from build123d import *

# Parameters (mm, degrees)
SKETCH1_W             = 50
SKETCH1_H             = 50
BOSS_EXTRUDE1_DEPTH   = 10
BOSS_EXTRUDE1_2_DEPTH = 10
BOSS_EXTRUDE2_DEPTH   = 50
SKETCH3_W             = 30
SKETCH3_H             = 30
CUT_EXTRUDE1_DEPTH    = 90
SKETCH4_W             = 10
SKETCH4_H             = 29.860616381
SKETCH4_H_2           = 30
CUT_EXTRUDE2_DEPTH    = 90
SKETCH5_W             = 50
SKETCH5_H             = 50
BOSS_EXTRUDE3_DEPTH   = 10
SKETCH6_R             = 12
CUT_EXTRUDE3_DEPTH    = 80
SKETCH13_W            = 50
SKETCH13_H            = 50
CUT_EXTRUDE5_DEPTH    = 160
SKETCH7_R             = 15.5
BOSS_EXTRUDE4_DEPTH   = 337.81
SKETCH14_W            = 50
SKETCH14_H            = 50
BOSS_EXTRUDE5_DEPTH   = 10
BOSS_EXTRUDE6_DEPTH   = 10
BOSS_EXTRUDE7_DEPTH   = 10
SKETCH17_R            = 15.5
CUT_EXTRUDE6_DEPTH    = 70
SKETCH19_R            = 12.7
CUT_EXTRUDE7_DEPTH    = 70
SKETCH20_R            = 12.7
BOSS_EXTRUDE11_DEPTH  = 10
SKETCH26_R            = 12
BOSS_EXTRUDE12_DEPTH  = 10
SKETCH27_R            = 13
CUT_EXTRUDE8_DEPTH    = 70


with BuildPart() as part:
    # Sketch1 → Boss-Extrude1 (new body)
    with BuildSketch(Plane.XY):
        with Locations((25, 25)):
            Rectangle(SKETCH1_W, SKETCH1_H)
    extrude(amount=BOSS_EXTRUDE1_DEPTH)

    # Sketch2 → Boss-Extrude2 (add)
    with BuildSketch(Plane(origin=(0, 0, 0), x_dir=(1, 0, 0), z_dir=(0, 1, 0))):
        with BuildLine():
            Line((0, 0), (50, 0))
            Line((50, 0), (50, 30))
            ThreePointArc((50, 30), (44.142135624, 44.142135624), (30, 50))
            Line((30, 50), (20, 50))
            ThreePointArc((20, 50), (5.857864376, 44.142135624), (0, 30))
            Line((0, 30), (0, 0))
        make_face()
    extrude(amount=BOSS_EXTRUDE2_DEPTH)

    # Sketch3 → Cut-Extrude1 (cut)
    with BuildSketch(Plane.XY.offset(10)):
        with Locations((25, 25)):
            Rectangle(SKETCH3_W, SKETCH3_H)
    extrude(amount=-CUT_EXTRUDE1_DEPTH, mode=Mode.SUBTRACT)

    # Sketch4 → Cut-Extrude2 (cut)
    with BuildSketch(Plane.XY.offset(10)):
        with Locations((45, 25.06969181)):
            Rectangle(SKETCH4_W, SKETCH4_H)
        with Locations((5, 25)):
            Rectangle(SKETCH4_W, SKETCH4_H_2)
    extrude(amount=-CUT_EXTRUDE2_DEPTH, mode=Mode.SUBTRACT)


with BuildPart() as body_2:
    # Sketch1 → Boss-Extrude1 2 (new body)
    with BuildSketch(Plane.XY):
        with Locations((25, -320)):
            Rectangle(SKETCH1_W, SKETCH1_H)
    extrude(amount=BOSS_EXTRUDE1_2_DEPTH)

    # Sketch13 → Cut-Extrude5 (cut)
    with BuildSketch(Plane(origin=(0, 0, 0), x_dir=(-1, 0, 0), z_dir=(0, 0, -1))):
        with Locations((-25, -320)):
            Rectangle(SKETCH13_W, SKETCH13_H)
    extrude(amount=-CUT_EXTRUDE5_DEPTH, mode=Mode.SUBTRACT)


with BuildPart() as cut_extrude2_piece_1:
    # of the separate pieces the step leaves, piece 1, a body of its own (cut_extrude2_pieces)
    add(part.part.solids().sort_by_distance((0, 0, 10))[0])



with BuildPart() as cut_extrude2_piece_2:
    # of the separate pieces the step leaves, piece 2, a body of its own (cut_extrude2_pieces)
    add(part.part.solids().sort_by_distance((0, 50, 10))[0])


with BuildPart() as cut_extrude2_piece_1_1:
    add(cut_extrude2_piece_1.part)

    add(cut_extrude2_piece_2.part)  # Boss-Extrude3 merges Cut-Extrude2 piece 2
    # Sketch5 → Boss-Extrude3 (add)
    with BuildSketch(Plane.XY.offset(10)):
        with Locations((25, 25)):
            Rectangle(SKETCH5_W, SKETCH5_H)
    extrude(amount=-BOSS_EXTRUDE3_DEPTH)

    # Sketch6 → Cut-Extrude3 (cut)
    with BuildSketch(Plane.XZ):
        with Locations(Location((25, -30, 0), (0, 0, 270))):
            Circle(SKETCH6_R)
    extrude(amount=-CUT_EXTRUDE3_DEPTH, mode=Mode.SUBTRACT)

    # Sketch7 → Boss-Extrude4 (add)
    with BuildSketch(Plane.XY.offset(10)):
        with Locations((25, 25)):
            Circle(SKETCH7_R)
    extrude(amount=BOSS_EXTRUDE4_DEPTH)

    # Sketch14 → Boss-Extrude5 (add)
    with BuildSketch(Plane.XY.offset(347.81)):
        with Locations((25, 25)):
            Rectangle(SKETCH14_W, SKETCH14_H)
    extrude(amount=BOSS_EXTRUDE5_DEPTH)

    # Sketch15 → Boss-Extrude6 (add)
    with BuildSketch(Plane(origin=(0, 50, 0), x_dir=(1, 0, 0), z_dir=(0, 1, 0))):
        with BuildLine():
            Line((0, -357.81), (50, -357.81))
            Line((50, -357.81), (50, -387.81))
            ThreePointArc((50, -387.81), (44.142135624, -401.952135624), (30, -407.81))
            Line((30, -407.81), (20, -407.81))
            ThreePointArc((20, -407.81), (5.857864376, -401.952135624), (0, -387.81))
            Line((0, -387.81), (0, -357.81))
        make_face()
    extrude(amount=-BOSS_EXTRUDE6_DEPTH)

    # Sketch16 → Boss-Extrude7 (add)
    with BuildSketch(Plane.XZ):
        with BuildLine():
            Line((0, 347.81), (50, 347.81))
            Line((50, 347.81), (50, 387.81))
            ThreePointArc((50, 387.81), (44.142135624, 401.952135624), (30, 407.81))
            Line((30, 407.81), (20, 407.81))
            ThreePointArc((20, 407.81), (5.857864376, 401.952135624), (0, 387.81))
            Line((0, 387.81), (0, 347.81))
        make_face()
    extrude(amount=-BOSS_EXTRUDE7_DEPTH)

    # Sketch17 → Cut-Extrude6 (cut)
    with BuildSketch(Plane.XZ):
        with Locations(Location((25, 387.81, 0), (0, 0, 270))):
            Circle(SKETCH17_R)
    extrude(amount=-CUT_EXTRUDE6_DEPTH, mode=Mode.SUBTRACT)

    # Sketch19 → Cut-Extrude7 (cut)
    with BuildSketch(Plane.XZ):
        with Locations(Location((32.852399557, -6.497982337, 0), (0, 0, 270))):
            Circle(SKETCH19_R)
    extrude(amount=-CUT_EXTRUDE7_DEPTH, mode=Mode.SUBTRACT)

    # Sketch20 → Boss-Extrude11 (add)
    with BuildSketch(Plane.XZ):
        with Locations((25, -30)):
            Circle(SKETCH20_R)
    extrude(amount=-BOSS_EXTRUDE11_DEPTH)

    # Sketch26 → Boss-Extrude12 (add)
    with BuildSketch(Plane(origin=(0, 50, 0), x_dir=(1, 0, 0), z_dir=(0, 1, 0))):
        with Locations((25, 30)):
            Circle(SKETCH26_R)
    extrude(amount=-BOSS_EXTRUDE12_DEPTH)

    # Sketch27 → Cut-Extrude8 (cut)
    with BuildSketch(Plane(origin=(0, 50, 0), x_dir=(1, 0, 0), z_dir=(0, 1, 0))):
        with Locations(Location((32.852399557, 6.497982337, 0), (0, 0, 270))):
            Circle(SKETCH27_R)
    extrude(amount=-CUT_EXTRUDE8_DEPTH, mode=Mode.SUBTRACT)


solid = cut_extrude2_piece_1_1.part
CAD build for the part. Positions are in the model's coordinates, mm. A direction names the side the tool comes from. Round coordinates to 2 decimals unless told otherwise and drop trailing zeros. Loops run counter-clockwise (first coordinate to the right, second up) from the corner with the lowest first, then second, coordinate; pieces in that order, holes last. Notation, with made-up numbers: (1, -3.5) - (44, -3.5) arc R14 cw to (44, 5.5) - close; hole circle Ø10 at (-16.5, 16). An arc over 180 degrees is marked (long way). Put each result on its own line as item: value.
1. 3-axis set-ups, long thin cutter, end or side, ignore diameter. For faces 4 (the flat face through (13.5, 36.5, 10)), 5 (the cylindrical face through (25.682, 44.93, 403.295)), 6 (the flat face through (25, 25, 357.81)): which of +Z, -Z, +X, -X, +Y, -Y reach the whole face in a straight line?
Geometry check:
face 4: none
face 5: +Y, -Y
face 6: +Z, +X, -X
2. Wall check: line 1 (Z direction, x = 9, y = 24); line 2 (Y direction, x = 21.5, z = 358); line 3 (X direction, y = 42, z = 387). Give the ranges that are in metal, low to high.
Geometry check:
line 1: 0 to 10, 347.81 to 357.81
line 2: 0 to 10, 40 to 50
line 3: 0 to 9.52, 40.48 to 50
3. Slice it at A-A on y = 25. List the corners of the cut face in (x, z).
Geometry check:
outline: (0, 0) - (21.59, 0) arc R13 cw to (44.11, 0) - (50, 0) - (50, 10) - (40.5, 10) - (40.5, 347.81) - (50, 347.81) - (50, 357.81) - (0, 357.81) - (0, 347.81) - (9.5, 347.81) - (9.5, 10) - (0, 10) - close
4. Slice it at B-B on z = 104. List the corners of the cut face in (x, y).
Geometry check:
outline: circle Ø31 at (25, 25)
5. Pin check, flat tips, straight feed: P1, Ø24, axis at x = 7.5, y = 26, coming from the -Z side; P2, Ø25, axis at x = 25.5, y = 13.5, coming from the +Z side; P3, Ø1.5, axis at y = 12.5, z = 100.5, coming from the -X side; P4, Ø18.5, axis at x = 25, z = 387.81, coming from the +Y side. Stop position of each tip, or through.
Geometry check:
P1: z = 0
P2: z = 407.81
P3: x = 14.89
P4: through
6. Two-plate mould, pull along Z, no slides. Class faces 1 (the flat face through (11, 25, 0)), 2 (the cylindrical face through (44.297, 45.07, 401.796)), 3 (the flat face through (13.5, 36.5, 347.81)): released by +Z, released by -Z, zero draft, split by the parting line, or undercut.
Geometry check:
face 1: released by -Z
face 2: released by +Z
face 3: undercut
